The model under review builds one solid part; all positions refer to its coordinate system, in mm. Coordinates: 2 decimals unless noted, no trailing zeros. Order: outer loops, then holes, each group sorted by start corner. A loop starts at its lowest first (then second) coordinate and runs counter-clockwise, first axis right, second up. Notation, with made-up numbers: (68.25, 69) - (79.25, 69) arc R31 cw to (79.25, 100) - close; hole circle Ø3 at (89, -1.75). An arc over 180 degrees is marked (long way). Answer in a Markdown table with one row per item.
Autodesk Inventor part; units mm, degrees
ref_plane "YZ Plane" through (0, 0, 0) normal (1, 0, 0) x (0, 1, 0)
ref_plane "XZ Plane" through (0, 0, 0) normal (0, 1, 0) x (-1, 0, 0)
ref_plane "XY Plane" through (0, 0, 0) normal (0, 0, 1) x (1, 0, 0)
sketch "Sketch1" plane through (0, 0, 0) normal (0, 0, 1) x (1, 0, 0)
  circle A0 centre (0, 0) radius 5
  circle A1 centre (0, 130) radius 5
  line L0 (-15, 145) -> (15, 145)
  line L1 (15, 145) -> (15, -15)
  line L2 (15, -15) -> (-15, -15)
  line L3 (-15, -15) -> (-15, 145)
  circle A2 centre (0, 130) radius 15
  circle A3 centre (0, 0) radius 15
  point P0 (15, 130)
  point P1 (-15, 130)
  point P2 (-15, 0)
  point P3 (15, 0)
  dimension "d0" = 10
  dimension "d1" = 10
  dimension "d2" = 130
  dimension "d3" = 30
  dimension "d4" = 15
  dimension "d5" = 15
  dimension "d6" = 15
  dimension "d7" = 30
  dimension "d8" = 30
sketch "Sketch2" plane through (0, 0, 0) normal (1, 0, 0) x (0, 1, 0)
  point P0 (0, 0)
extrude "Extrusion1" add sketch "Sketch1" along normal blind 3 contours A2 | A2 L1 A3 L3 | A3
sketch "Sketch3" plane through (0, 0, 3) normal (0, 0, 1) x (1, 0, 0)
  circle A0 centre (-10, 97) radius 1.5
  line L0 (-15, 130) -> (-15, 0)
  circle A1 centre (0, 130) radius 5
  point P0 (0, 0)
  dimension "d11" = 3
  dimension "d12" = 5
  dimension "d13" = 33
extrude "Extrusion2" cut sketch "Sketch3" against normal blind 3 contours A0
properties part number "Link3Do"
Item 1: Clearance check with flat-ended pins moving along their axes: pin 1 Ø9 at (x, y) = (0, 0) entering from -Z; pin 2 Ø1 at (x, z) = (-1.5, 1) entering from -Y. State where each tip first meets the part, or that it passes through.
Check values:
| item | result |
|---|---|
| pin 1 | through |
| pin 2 | y = -14.97 |
Item 2: We need section B-B, the plane x = 0. Write out the cut boundary in (y, z).
Check values:
| item | result |
|---|---|
| outline | (-15, 0) - (-5, 0) - (-5, 3) - (-15, 3) - close; (5, 0) - (125, 0) - (125, 3) - (5, 3) - close; (135, 0) - (145, 0) - (145, 3) - (135, 3) - close |
Item 3: Mouldability with a two-part tool opening along Y and no side actions: class faces 1 (the face through (15, 66, 1)), 2 (the face through (0, -15, 1)), 3 (the face through (0, 145, 1)), 4 (the face through (2.307, 134.436, 1.479)) as +Y half, -Y half, draft (parallel to the pull), parting line (faces both ways), or undercut.
Check values:
| item | result |
|---|---|
| face 1 | draft |
| face 2 | -Y half |
| face 3 | +Y half |
| face 4 | undercut |
Item 4: We need section D-D, the plane x = -10. Write out the cut boundary in (y, z), then the cut area to 3 significant figures.
Check values:
| item | result |
|---|---|
| outline | (-11.18, 0) - (95.5, 0) - (95.5, 3) - (-11.18, 3) - close; (98.5, 0) - (141.18, 0) - (141.18, 3) - (98.5, 3) - close |
| area | 448 mm^2 |
Item 5: To check wall thickness, follow line 1 (Y direction, x = 0, z = 0.75); line 2 (Y direction, x = -4.25, z = 2.1); line 3 (X direction, y = 1, z = 0.45). State the ranges of each line that lie inside material, in increasing order. Write a range as from..to.
Check values:
| item | result |
|---|---|
| line 1 | -15..-5, 5..125, 135..145 |
| line 2 | -14.39..-2.63, 2.63..127.37, 132.63..144.39 |
| line 3 | -15..-4.9, 4.9..15 |
Item 6: We need section A-A, the plane y = 97. Write out the cut boundary in (x, z), then the cut area to 3 significant figures.
Check values:
| item | result |
|---|---|
| outline | (-15, 0) - (-11.5, 0) - (-11.5, 3) - (-15, 3) - close; (-8.5, 0) - (15, 0) - (15, 3) - (-8.5, 3) - close |
| area | 81.0 mm^2 |
Item 7: We need section C-C, the plane z = 2.35. Write out the cut boundary in (x, y), then the cut area to 3 significant figures.
Check values:
| item | result |
|---|---|
| outline | (-15, 0) arc R15 ccw to (15, 0) - (15, 130) arc R15 ccw to (-15, 130) - close; hole circle Ø3 at (-10, 97); hole circle Ø10 at (0, 0); hole circle Ø10 at (0, 130) |
| area | 4,440 mm^2 |
